Geometry: see drawing. Coordinates: mm, zero at the bounding-box minimum. Coordinates: 2 decimals unless noted, no trailing zeros. Order: outer loops, then holes, each group sorted by start corner. A loop starts at its lowest first (then second) coordinate and runs counter-clockwise, first axis right, second up. Notation, with made-up numbers: (3, -1) - (48, -1) arc R17 cw to (48, 23) - close; hole circle Ø8 at (32, 28). An arc over 180 degrees is marked (long way). Use a Markdown table: item, result. Add a question column.
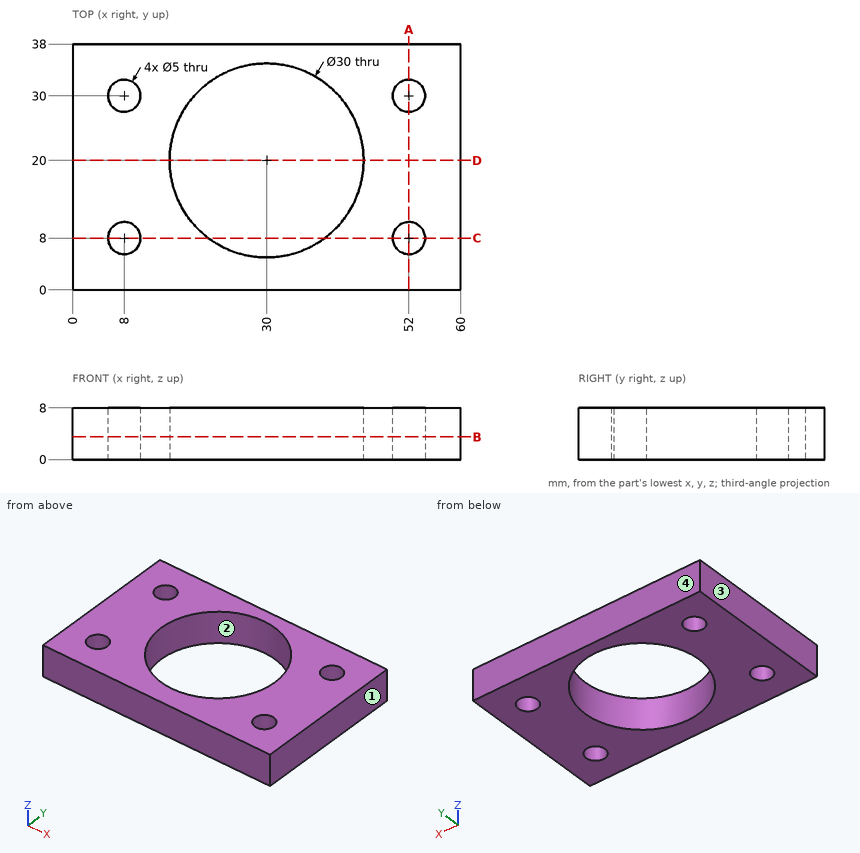
1) Section query C-C (y = 8). Return the cut outline in (x, z).
2) Section query A-A (x = 52). Return the cut outline in (y, z).
3) Section query B-B (z = 3.5). Return the cut outline in (x, y), and give its area (3 significant figures).
4) Section query D-D (y = 20). Return the cut outline in (x, z), and give its area (3 significant figures).
5) Line query: line 1 (Y direction, x = 8, z = 6.25); line 2 (X direction, y = 20, z = 2); line 3 (X direction, y = 8, z = 3.25). Output: solid intervals per line, ascending. Write a range as from..to.
6) Draft query along X for the marked faces 1, 2, 3 and 4. Return one class per face: released by +X, released by -X, zero draft, split by the parting line, or undercut.
From the geometry:
| question | item | result |
|---|---|---|
| 1 | outline | (0, 0) - (5.5, 0) - (5.5, 8) - (0, 8) - close; (10.5, 0) - (21, 0) - (21, 8) - (10.5, 8) - close; (39, 0) - (49.5, 0) - (49.5, 8) - (39, 8) - close; (54.5, 0) - (60, 0) - (60, 8) - (54.5, 8) - close |
| 2 | outline | (0, 0) - (5.5, 0) - (5.5, 8) - (0, 8) - close; (10.5, 0) - (27.5, 0) - (27.5, 8) - (10.5, 8) - close; (32.5, 0) - (38, 0) - (38, 8) - (32.5, 8) - close |
| 3 | outline | (0, 0) - (60, 0) - (60, 38) - (0, 38) - close; hole circle Ø5 at (8, 8); hole circle Ø5 at (8, 30); hole circle Ø30 at (30, 20); hole circle Ø5 at (52, 8); hole circle Ø5 at (52, 30) |
| 3 | area | 1,490 mm^2 |
| 4 | outline | (0, 0) - (15, 0) - (15, 8) - (0, 8) - close; (45, 0) - (60, 0) - (60, 8) - (45, 8) - close |
| 4 | area | 240 mm^2 |
| 5 | line 1 | y = 0..5.5, 10.5..27.5, 32.5..38 |
| 5 | line 2 | x = 0..15, 45..60 |
| 5 | line 3 | x = 0..5.5, 10.5..21, 39..49.5, 54.5..60 |
| 6 | face 1 | released by +X |
| 6 | face 2 | undercut |
| 6 | face 3 | released by -X |
| 6 | face 4 | zero draft |
